Work out the finished part from the listing and answer in its coordinate system (mm). A direction names the side the tool comes from. Coordinates: 2 decimals unless noted, no trailing zeros. Loops run counter-clockwise (first coordinate to the right, second up) from the corner with the lowest first, then second, coordinate; pieces in that order, holes last. Notation, with made-up numbers: (-19, -13.75) -> (27, -13.75) arc R28 ccw to (27, 9.25) -> close; hole circle Ø1 at (68.25, -10). An arc over 180 degrees is marked (long way). One line per question, with ' | ' between items.
```python
from build123d import *

# Parameters (mm, degrees)
SKETCH1_W               = 30
SKETCH1_H               = 16
BOSS_EXTRUDE1_DEPTH     = 14
SKETCH3_R               = 9.955
BOSS_EXTRUDE2_DEPTH     = 30
SKETCH4_W               = 11.4
SKETCH4_H               = 3
CUT_EXTRUDE1_DEPTH      = 30
SKETCH5_R               = 5
CUT_EXTRUDE2_DEPTH      = 15
CUT_EXTRUDE5_DEPTH      = 15
SKETCH7_R               = 2
SKETCH7_W               = 7.475303805
SKETCH7_H               = 1
CUT_EXTRUDE7_DEPTH      = 1
CUT_EXTRUDE7_DEPTH_BACK = 3
SKETCH7_4_R             = 2
CUT_EXTRUDE9_DEPTH      = 18.955
SKETCH11_R              = 3.5
CUT_EXTRUDE10_DEPTH     = 0.93


with BuildPart() as part:
    # Sketch1 → Boss-Extrude1 (new body)
    with BuildSketch(Plane(origin=(0, 0, 0), x_dir=(0, 0, -1), z_dir=(1, 0, 0))):
        with Locations((0.927835052, 0.737113402)):
            Rectangle(SKETCH1_W, SKETCH1_H)
    extrude(amount=-BOSS_EXTRUDE1_DEPTH)

    # Sketch3 → Boss-Extrude2 (add)
    with BuildSketch(Plane(origin=(0, 0, -15.927835052), x_dir=(-1, 0, 0), z_dir=(0, 0, -1))):
        with Locations((14, 0.737113402)):
            Circle(SKETCH3_R)
    extrude(amount=-BOSS_EXTRUDE2_DEPTH)

    # Sketch4 → Cut-Extrude1 (cut)
    with BuildSketch(Plane(origin=(0, 0, -15.927835052), x_dir=(-1, 0, 0), z_dir=(0, 0, -1))):
        with Locations((5.7, 0.737113402)):
            Rectangle(SKETCH4_W, SKETCH4_H)
    extrude(amount=-CUT_EXTRUDE1_DEPTH, mode=Mode.SUBTRACT)

    # Sketch5 → Cut-Extrude2 (cut)
    with BuildSketch(Plane.XY.offset(14.072164948)):
        with Locations((-13.955, 0.737113402)):
            Circle(SKETCH5_R)
    extrude(amount=-CUT_EXTRUDE2_DEPTH, mode=Mode.SUBTRACT)

    # Sketch6 → Cut-Extrude5 (cut)
    with BuildSketch(Plane(origin=(0, 0, -15.927835052), x_dir=(-1, 0, 0), z_dir=(0, 0, -1))):
        with BuildLine():
            Line((16, 2.987113402), (16, -1.512886598))
            ThreePointArc((16, -1.512886598), (11.015686517, 0.737113402), (16, 2.987113402))
        make_face()
    extrude(amount=-CUT_EXTRUDE5_DEPTH, mode=Mode.SUBTRACT)

    # Sketch7 → Cut-Extrude7 (cut, two sides)
    with BuildSketch(Plane.XZ.offset(7.262886598)) as cut_extrude7_sk:
        Polygon((-6.074118703, 3.222164948), (-3.1729336, 4.897164948), (-3.1729336, 8.247164948), (-6.074118703, 9.922164948), (-8.975303805, 8.247164948), (-8.975303805, 4.897164948), align=None)
        with Locations((-6.074118703, 6.572164948)):
            Circle(SKETCH7_R, mode=Mode.SUBTRACT)
        Polygon((-6.074118703, -11.777835052), (-3.1729336, -10.102835052), (-3.1729336, -6.752835052), (-6.074118703, -5.077835052), (-8.975303805, -6.752835052), (-8.975303805, -10.102835052), align=None)
        with Locations((-5.237651903, -0.927835052)):
            Rectangle(SKETCH7_W, SKETCH7_H)
    extrude(amount=CUT_EXTRUDE7_DEPTH, mode=Mode.SUBTRACT)
    extrude(cut_extrude7_sk.sketch, amount=-CUT_EXTRUDE7_DEPTH_BACK, mode=Mode.SUBTRACT)

    # Sketch7_4 → Cut-Extrude9 (cut, through all)
    with BuildSketch(Plane.XZ.offset(7.262886598)):
        with Locations((-6.074118703, -8.427835052)):
            Circle(SKETCH7_4_R)
        with Locations((-6.074118703, 6.572164948)):
            Circle(SKETCH7_4_R)
    extrude(amount=-CUT_EXTRUDE9_DEPTH, mode=Mode.SUBTRACT)

    # Sketch11 → Cut-Extrude10 (cut)
    with BuildSketch(Plane(origin=(0, 8.737113402, 0), x_dir=(1, 0, 0), z_dir=(0, 1, 0))):
        with Locations((-6.074118703, -6.572164948)):
            Circle(SKETCH11_R)
        with Locations((-6.074118703, 8.427835052)):
            Circle(SKETCH11_R)
    extrude(amount=CUT_EXTRUDE10_DEPTH, mode=Mode.SUBTRACT)


solid = part.part
```
1) Flat-ended cylindrical pins translate along their axes: pin 1 (10.5 mm diameter, centred on x = -2.5, z = 1, fed in from +Y); pin 2 (4.5 mm diameter, centred on x = -6.07, z = 6.57, fed in from -Y); pin 3 (5.5 mm diameter, centred on x = -7, z = -8, fed in from +Y). Find the tip coordinate at first contact, or state that the pin passes through.
Check values:
pin 1: stops at y = 8.74 | pin 2: stops at y = -4.26 | pin 3: stops at y = 9.74
2) Find section B-B (z = -3). Write down the section's boundary in (x, y) (3 decimals), plus the area to 3 significant figures.
Check values:
outline: (-16, -1.513) -> (-16, 2.987) arc R3 cw to (-11.4, 2.206) -> (-11.4, 2.237) -> (0, 2.237) -> (0, 8.737) -> (-8.075, 8.737) arc R9.955 ccw (long way) to (-8.075, -7.263) -> (0, -7.263) -> (0, -0.763) -> (-11.4, -0.763) -> (-11.4, -0.732) arc R3 cw to start | area: 337 mm^2
3) Find section A-A (x = -10.5). Write down the section's boundary in (y, z).
Check values:
outline: (-8.58, -15.93) -> (-0.76, -15.93) -> (-0.76, -0.93) -> (-2.88, -0.93) -> (-2.88, 14.07) -> (-8.58, 14.07) -> close; (2.24, -15.93) -> (10.06, -15.93) -> (10.06, 14.07) -> (4.35, 14.07) -> (4.35, -0.93) -> (2.24, -0.93) -> close
4) For faces 4 (the face through (-6, 2.237, -1)), 5 (the face through (-16.3, 0.8, -0.928)), 6 (the face through (-13.48, 3.69, -8.53)), 7 (the face through (-9.574, 9.087, -8.475)), 8 (the face through (-3.173, -6, 7)), determine the directions among +Z, -Z, +X, -X, +Y, -Y from which every point of the face is accessible in a straight line to the end or side of a thin tool.
Check values:
face 4: +Z, -Z, +X | face 5: +Z | face 6: +Z, -Z | face 7: +X, +Y | face 8: -Y
5) Find the intervals of material crossed by line 1 along Y through (x, z) = (-1.75, 4.5); line 2 along X through (y, z) = (4.5, 6); line 3 along Z through (x, y) = (-16.25, 3.75), in increasing order.
Check values:
line 1: y = -7.26 to -0.76, 2.24 to 8.74 | line 2: x = -23.22 to -17.25, -10.66 to -7.99, -4.16 to 0 | line 3: z = -15.93 to -0.93
6) Find section C-C (z = 1). Write down the section's boundary in (x, y) (3 decimals), plus the area to 3 significant figures.
Check values:
outline: (-9.185, -0.763) arc R5 cw (long way) to (-9.185, 2.237) -> (0, 2.237) -> (0, 8.737) -> (-8.075, 8.737) arc R9.955 ccw (long way) to (-8.075, -7.263) -> (0, -7.263) -> (0, -0.763) -> close | area: 290 mm^2
7) The mould has two halves that part along Z. Classify faces 1 (the face through (-11.8, 3.1, -15.928)), 2 (the face through (-6, -0.763, -1)), 3 (the face through (-5, -2.54, -6.74)): released by +Z, released by -Z, zero draft, split by the parting line, or undercut.
Check values:
face 1: released by -Z | face 2: zero draft | face 3: undercut
8) Find section D-D (x = -14). Write down the section's boundary in (y, z), plus the area to 3 significant figures.
Check values:
outline: (-9.22, -15.93) -> (-2.26, -15.93) -> (-2.26, -0.93) -> (-4.26, -0.93) -> (-4.26, 14.07) -> (-9.22, 14.07) -> close; (3.74, -15.93) -> (10.69, -15.93) -> (10.69, 14.07) -> (5.74, 14.07) -> (5.74, -0.93) -> (3.74, -0.93) -> close | area: 357 mm^2
